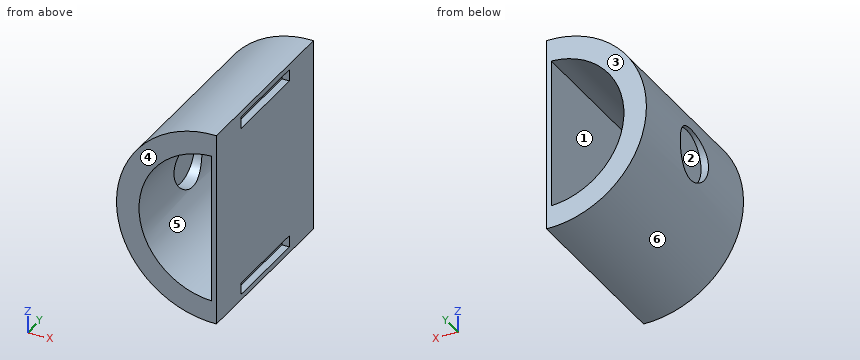
from build123d import *

# Parameters (mm, degrees)
SKETCH1_R                = 130
BOSS_EXTRUDE1_DEPTH      = 241.01
SKETCH2_R                = 100
CUT_EXTRUDE1_DEPTH       = 304.126739335
BOSS_EXTRUDE2_DEPTH      = 241.01
BODY_DELETE_KEEP_1_DEPTH = 241.01
SKETCH8_R                = 35
CUT_EXTRUDE2_DEPTH       = 10
CUT_EXTRUDE9_DEPTH       = 10
CUT_EXTRUDE9_DEPTH_BACK  = 10
SKETCH10_R               = 35
SKETCH16_W               = 15.74894652
SKETCH16_H               = 120.505
CUT_EXTRUDE10_DEPTH      = 10


# Read off the part's stored shape, not the designer's step: Body-Delete/Keep 1
with BuildPart() as part:
    # Sketch1 → Boss-Extrude1 (new body)
    with BuildSketch(Plane(origin=(0, 0, 0), x_dir=(1, 0, 0), z_dir=(0, 1, 0))):
        with Locations(Location((0, 0, 0), (0, 0, 270))):
            Circle(SKETCH1_R)
    extrude(amount=BOSS_EXTRUDE1_DEPTH)

    # Sketch2 → Cut-Extrude1 (cut, through all)
    with BuildSketch(Plane(origin=(0, 241.01, 0), x_dir=(1, 0, 0), z_dir=(0, 1, 0))):
        with Locations(Location((0, 0, 0), (0, 0, 270))):
            Circle(SKETCH2_R)
    extrude(amount=-CUT_EXTRUDE1_DEPTH, mode=Mode.SUBTRACT)


with BuildPart() as body_2:
    # Sketch5 → Boss-Extrude2 (new body)
    with BuildSketch(Plane(origin=(0, 0, 0), x_dir=(1, 0, 0), z_dir=(0, 1, 0))):
        Polygon((-3.175, -0.773064833), (-3.175, 104.496382322), (3.175, 104.496382322), (3.175, 0), (3.175, -106.678671161), (-3.175, -106.678671161), align=None)
    extrude(amount=BOSS_EXTRUDE2_DEPTH)


with BuildPart() as body_3:
    # Split1: the piece on the far side of the plane
    add(part.part)
    split(bisect_by=Plane(origin=(3.175, 0, 0), x_dir=(0, 0, 1), z_dir=(1, 0, 0)), keep=Keep.BOTTOM)

    # Combine2: union body 2
    add(body_2.part)

    # Sketch8 → Cut-Extrude2 (cut)
    with BuildSketch(Plane(origin=(-130, 0, 0), x_dir=(0, 0, -1), z_dir=(1, 0, 0))):
        with Locations(Location((0, 121.833368443, 0), (0, 0, 180))):
            Circle(SKETCH8_R)
    extrude(amount=CUT_EXTRUDE2_DEPTH, mode=Mode.SUBTRACT)

    # Sketch10 → Cut-Extrude9 (cut, two sides: drawn at the far end of the back side and taken through both)
    with BuildSketch(Plane(origin=(-100, 0, 0), x_dir=(0, 0, -1), z_dir=(1, 0, 0)).offset(-CUT_EXTRUDE9_DEPTH_BACK)):
        with Locations(Location((0, 121.833368443, 0), (0, 0, 180))):
            Circle(SKETCH10_R)
    extrude(amount=CUT_EXTRUDE9_DEPTH + CUT_EXTRUDE9_DEPTH_BACK, mode=Mode.SUBTRACT)

    # Sketch16 → Cut-Extrude10 (cut)
    with BuildSketch(Plane(origin=(3.175, 0, 0), x_dir=(0, 0, -1), z_dir=(1, 0, 0))):
        with Locations((-114.583839718, 121.169184221)):
            Rectangle(SKETCH16_W, SKETCH16_H)
    cut_extrude10 = extrude(amount=-CUT_EXTRUDE10_DEPTH, mode=Mode.SUBTRACT)

    # Mirror1: Cut-Extrude10 across plane
    add(cut_extrude10.mirror(Plane.XY), mode=Mode.SUBTRACT)


with BuildPart() as part_1:
    add(part.part)

    # Split1
    split(bisect_by=Plane(origin=(3.175, 0, 0), x_dir=(0, 0, 1), z_dir=(1, 0, 0)), keep=Keep.TOP)

    # Body-Delete/Keep 1 outline → Body-Delete/Keep 1 (cut)
    with BuildSketch(Plane(origin=(0, 0, 0), x_dir=(1, 0, 0), z_dir=(0, 1, 0))):
        with BuildLine():
            ThreePointArc((3.175, -129.961222582), (130, 0), (3.175, 129.961222582))
            Line((3.175, 129.961222582), (3.175, 99.949584166))
            ThreePointArc((3.175, 99.949584166), (100, 0), (3.175, -99.949584166))
            Line((3.175, -99.949584166), (3.175, -129.961222582))
        make_face()
    extrude(amount=BODY_DELETE_KEEP_1_DEPTH, mode=Mode.SUBTRACT)


solid = body_3.part
The model under review builds one solid part; all positions refer to its coordinate system, in mm. Face numbers are marked on the shaded views. A direction names the side the tool comes from. Give positions to 0.01 mm unless a question says otherwise; leave off trailing zeros. Loops run counter-clockwise (first coordinate to the right, second up) from the corner with the lowest first, then second, coordinate; pieces in that order, holes last. Notation, with made-up numbers: (33, -7.75) -> (44, -7.75) arc R16 cw to (44, 15.25) -> close; hole circle Ø4 at (26.5, -23.75). An arc over 180 degrees is marked (long way). Answer as a JSON object with one key per item and string values. Group by question number.
Q1. Take a section at D-D (x = -40.5). Write out the cut boundary in (y, z), plus the area to 3 significant figures.
Q2. Draft analysis for pull direction Z (two halves, no side actions). For the marked faces 4, 5 and 6, state which applies: pulls with the +Z half, pulls with the -Z half, needs draft (parallel to the pull), parting line crosses it, or undercut.
Q3. Take a section at A-A (y = 67.5). Write out the cut boundary in (x, z) (3 decimals), plus the area to 3 significant figures.
Q4. Insertion check: pin 1 (5 mm diameter, centred on x = 0, y = 125, fed in from +Z); pin 2 (10 mm diameter, centred on y = 190, z = -73.5, fed in from -X); pin 3 (8 mm diameter, centred on x = -63, y = 81.5, fed in from -Z). Each pin has a flat end and moves straight along its axis. Give the tip position at first contact, or say it passes through.
Q5. Take a section at B-B (z = 0). Write out the cut boundary in (x, y) (3 decimals).
Q6. Wall thickness on line 1 along X through (y, z) = (129.5, -11.5) (3 decimals); line 2 along X through (y, z) = (208, 0.5) (3 decimals); line 3 along Y through (x, z) = (-127, 0): over which ranges is each line inside the solid? List them lowest first.
Q7. Tool access review of the marked faces 1, 2 and 3: name each direction out of +Z, -Z, +X, -X, +Y, -Y from which nothing blocks a thin tool from reaching the whole face with its end or side.
Q8. Take a section at C-C (x = 0). Write out the cut boundary in (y, z).
Answer below:
{
 "1": {"outline": "(0, -123.53) -> (241.01, -123.53) -> (241.01, -91.43) -> (0, -91.43) -> close; (0, 91.43) -> (241.01, 91.43) -> (241.01, 123.53) -> (0, 123.53) -> close", "area": "15,500 mm2"},
 "2": {"face 4": "needs draft", "face 5": "undercut", "face 6": "parting line crosses it"},
 "3": {"outline": "(-6.825, -122.458) -> (-6.825, -106.709) -> (3.175, -106.709) -> (3.175, 106.709) -> (-6.825, 106.709) -> (-6.825, 122.458) -> (3.175, 122.458) -> (3.175, 129.961) arc R130 ccw (long way) to (3.175, -129.961) -> (3.175, -122.458) -> close; hole (-3.175, -99.95) -> (-3.175, 99.95) arc R100 ccw to start", "area": "12,000 mm2"},
 "4": {"pin 1": "stops at z = 130", "pin 2": "stops at x = -110.49", "pin 3": "stops at z = -115.84"},
 "5": {"outline": "(-130, 0) -> (-100, 0) -> (-100, 86.833) -> (-110, 86.833) -> (-110, 156.833) -> (-100, 156.833) -> (-100, 241.01) -> (-130, 241.01) -> (-130, 156.833) -> (-120, 156.833) -> (-120, 86.833) -> (-130, 86.833) -> close; (-3.175, 0) -> (3.175, 0) -> (3.175, 241.01) -> (-3.175, 241.01) -> close"},
 "6": {"line 1": "x = -120 to -110, -3.175 to 3.175", "line 2": "x = -129.999 to -99.999, -3.175 to 3.175", "line 3": "y = 0 to 86.83, 156.83 to 241.01"},
 "7": {"face 1": "+Y, -Y", "face 2": "-X", "face 3": "+Z, -Z, +X, -X, +Y"},
 "8": {"outline": "(0, -130) -> (241.01, -130) -> (241.01, 130) -> (0, 130) -> close; hole (60.92, -122.46) -> (181.42, -122.46) -> (181.42, -106.71) -> (60.92, -106.71) -> close; hole (60.92, 106.71) -> (181.42, 106.71) -> (181.42, 122.46) -> (60.92, 122.46) -> close"}
}
